from build123d import *

# Parameters (mm, degrees)
F0_R     = 3.7719
F1_DEPTH = 228.6
F2_W     = 11.176
F2_H     = 4.3434
F3_DEPTH = 17.78
F5_D     = 5.334


with BuildPart() as f1:
    # F0 (on Top) → F1 (new body)
    with BuildSketch(Plane.XY):
        Circle(F0_R)
    extrude(amount=F1_DEPTH)

    # F2 (on face) → F3 (join)
    with BuildSketch(Plane.XY.offset(228.6)):
        Rectangle(F2_W, F2_H)
    extrude(amount=F3_DEPTH)

    # F5 (through all)
    with Locations(Plane(origin=(0, 2.1717, 0), x_dir=(-1, 0, 0), z_dir=(0, 1, 0))):
        with Locations((0, 237.998)):
            Hole(F5_D / 2)


solid = f1.part
Read the model definition and answer for the solid it produces. Units are mm, in the model's axes. A direction names the side the tool comes from. Give positions to 0.01 mm unless a question says otherwise; leave off trailing zeros. Write each loop counter-clockwise with the first axis right and the second up, starting at its lowest first coordinate (ties: lowest second). Pieces come first, ordered by that corner, then holes. Notation, with made-up numbers: (-37.5, 74.25) -> (-27.5, 74.25) arc R33 ccw to (-27.5, 107.25) -> close; hole circle Ø2 at (-29, 48.25). An arc over 180 degrees is marked (long way). Answer as a JSON object with one key per item and string values. Group by question number.
1) Find section A-A (x = 0). Write down the section's boundary in (y, z) (3 decimals), and give its area (3 significant figures).
2) Find section C-C (z = 220). Write down the section's boundary in (x, y).
3) Each of these flat-tipped pins is pushed along its axis until it touches: P1, Ø5.5, axis at x = -2, z = 234.5, coming from the -Y side; P2, Ø1.3, axis at x = 5, y = -0.5, coming from the -Z side; P3, Ø0.8, axis at x = 1, y = 3, coming from the +Z side; P4, Ø1, axis at x = -4.5, z = 28.5, coming from the -Y side. Where does it stop, or does it pass through?
4) A tool of negligible diameter and unlimited length cuts with its end or side. For faces 5 (the flat face through (5.588, 0, 237)), 6 (the flat face through (-1, -2.172, 235)), 7 (the flat face through (-1, 2.172, 235)), from which of +Z, -Z, +X, -X, +Y, -Y can it reach the whole face along a straight path? Write none if from no direction.
5) Consider L1, parallel to Z at x = 0, y = -0.75 (3 decimals); L2, parallel to Z at x = -0.5, y = -1.5; L3, parallel to Z at x = -3.5, y = 1.5. Determine where each line is inside the solid, lowest interval first. Write a range as from..to.
6) Find section B-B (y = 0). Write down the section's boundary in (x, z).
7) The mould has two halves that part along X. Classify faces 1 (the cylindrical face through (-0.35, -0.03, 240.64)), 2 (the cylindrical face through (-2.99, -2.3, 112.7)), 3 (the flat face through (0, 0, 0)), 4 (the flat face through (-5.588, 0, 237)): +X half, -X half, draft (parallel to the pull), parting line (faces both ways), or undercut.
Values follow:
{
 "1": {"outline": "(-3.772, 0) -> (3.772, 0) -> (3.772, 228.6) -> (2.172, 228.6) -> (2.172, 235.331) -> (-2.172, 235.331) -> (-2.172, 228.6) -> (-3.772, 228.6) -> close; (-2.172, 240.665) -> (2.172, 240.665) -> (2.172, 246.38) -> (-2.172, 246.38) -> close", "area": "1,780 mm2"},
 "2": {"outline": "circle Ø7.54 at (0, 0)"},
 "3": {"P1": "stops at y = -2.17", "P2": "stops at z = 228.6", "P3": "stops at z = 228.6", "P4": "passes through"},
 "4": {"face 5": "+Z, -Z, +X, +Y, -Y", "face 6": "+Z, +X, -X, -Y", "face 7": "+Z, +X, -X, +Y"},
 "5": {"L1": "z = 0..235.331, 240.665..246.38", "L2": "z = 0..235.38, 240.62..246.38", "L3": "z = 228.6..246.38"},
 "6": {"outline": "(-5.59, 228.6) -> (-3.77, 228.6) -> (-3.77, 0) -> (3.77, 0) -> (3.77, 228.6) -> (5.59, 228.6) -> (5.59, 246.38) -> (-5.59, 246.38) -> close; hole circle Ø5.33 at (0, 238)"},
 "7": {"face 1": "undercut", "face 2": "parting line", "face 3": "draft", "face 4": "-X half"}
}
